from build123d import *

# Parameters (mm, degrees)
F1_DEPTH  = 55
F2_R      = 8
F3_W      = 90
F3_H      = 90
F4_DEPTH  = 15
F5_R      = 8
F6_W      = 15
F6_H      = 10
F7_DEPTH  = 45
F8_R      = 5
F9_W      = 50
F9_H      = 45
F10_DEPTH = 50
F12_DEPTH = 45
F13_W     = 5
F13_H     = 40
F14_DEPTH = 15.001
F16_DEPTH = 5


with BuildPart() as f1:
    # F0 (on Front) → F1 (new body)
    with BuildSketch(Plane.XZ):
        Polygon((0, 18), (0, 0), (70, 0), (70, 45), (50, 45), (50, 20), (30, 20), (30, 45), (10, 45), (2.765372, 18), align=None)
    extrude(amount=-F1_DEPTH)

    # F2
    f2_edges = [f1.edges().sort_by_distance(p)[0] for p in [
        (30, 27.5, 20),
        (50, 27.5, 20),
    ]]
    fillet(f2_edges, radius=F2_R)

    # F3 (on face) → F4 (join)
    with BuildSketch(Plane(origin=(0, 0, 0), x_dir=(1, 0, 0), z_dir=(0, 0, -1))):
        with Locations((35, -25)):
            Rectangle(F3_W, F3_H)
    extrude(amount=F4_DEPTH)

    # F5
    f5_edges = [f1.edges().sort_by_distance(p)[0] for p in [
        (-10, 70, -7.5),
        (80, 70, -7.5),
        (-10, -20, -7.5),
        (80, -20, -7.5),
    ]]
    fillet(f5_edges, radius=F5_R)

    # F6 (on face) → F7 (join, through all)
    with BuildSketch(Plane.XY.offset(45)):
        with Locations((17.5, 60)):
            Rectangle(F6_W, F6_H)
    extrude(amount=-F7_DEPTH)

    # F8
    f8_edges = [f1.edges().sort_by_distance(p)[0] for p in [
        (25, 65, 22.5),
        (10, 65, 22.5),
    ]]
    fillet(f8_edges, radius=F8_R)

    # F9 (on face) → F10 (cut)
    with BuildSketch(Plane.XY.offset(45)):
        with Locations((40, 27.5)):
            Rectangle(F9_W, F9_H)
    extrude(amount=-F10_DEPTH, mode=Mode.SUBTRACT)

    # F11 (on face) → F12 (join)
    with BuildSketch(Plane.XY.offset(-5)):
        with BuildLine():
            Line((30, 50), (15, 50))
            Line((15, 50), (15, 35))
            ThreePointArc((15, 35), (25.606602, 39.393398), (30, 50))
        make_face()
    extrude(amount=F12_DEPTH)

    # F13 (on face) → F14 (cut, through all)
    with BuildSketch(Plane.XY):
        with Locations((-7.5, 35)):
            Rectangle(F13_W, F13_H)
        with Locations((77.5, 15)):
            Rectangle(F13_W, F13_H)
    extrude(amount=-F14_DEPTH, mode=Mode.SUBTRACT)

    # F15 (on face) → F16 (cut)
    with BuildSketch(Plane(origin=(0, 0, -15), x_dir=(1, 0, 0), z_dir=(0, 0, -1))):
        Polygon((0, 5), (60, -65), (60, 5), align=None)
    extrude(amount=-F16_DEPTH, mode=Mode.SUBTRACT)


solid = f1.part
Source: CAD feature listing. Evaluate the final solid. Frame: model axes, mm. A direction names the side the tool comes from. Coordinates: 2 decimals unless noted, no trailing zeros. Loops run counter-clockwise (first coordinate to the right, second up) from the corner with the lowest first, then second, coordinate; pieces in that order, holes last. Notation, with made-up numbers: (2, 57) - (16, 57) arc R18 ccw to (16, 83) - close; hole circle Ø6 at (8.25, 28). An arc over 180 degrees is marked (long way). One line per question, with ' | ' between items.
1) Set-up query: faces 1 (the face through (75, 15, -7)), 2 (the face through (6, 55, 18)), 3 (the face through (50, 52, 37)). Return all of +Z, -Z, +X, -X, +Y, -Y with unobstructed straight access to the full face (end or side cutting, diameter ignored); none if empty.
Report:
face 1: +Z, -Z, +X | face 2: +Z, -X, +Y | face 3: +Z, +Y, -Y
2) First-contact query: P1, Ø4, axis at x = -6.5, z = -9, coming from the -Y side; P2, Ø5, axis at y = 52.5, z = 33, coming from the -X side; P3, Ø4.5, axis at x = 24.5, y = 39, coming from the +Z side. Flat tips, straight axial feed; report the tip coordinate or a pass-through.
Report:
P1: stops at y = -19.6 | P2: stops at x = 6.11 | P3: stops at z = 40
3) Line query: line 1 along Y through (x, z) = (59.5, 18); line 2 along Y through (x, z) = (61, -4.5); line 3 along X through (y, z) = (22, 0.5). Output: solid intervals per line, ascending.
Report:
line 1: y = 0 to 5, 50 to 55 | line 2: y = -20 to 5, 50 to 70 | line 3: x = 0 to 15, 65 to 70
4) Section B-B, the plane x = 67.5. Return loops of the section in (y, z).
Report:
outline: (-20, -15) - (70, -15) - (70, 0) - (55, 0) - (55, 45) - (0, 45) - (0, 0) - (-20, 0) - close
5) Section C-C, the plane z = -1.5. Return loops of the section in (x, y).
Report:
outline: (-10, -12) arc R8 ccw to (-2, -20) - (72, -20) arc R8 ccw to (80, -12) - (80, -5) - (75, -5) - (75, 35) - (80, 35) - (80, 62) arc R8 ccw to (72, 70) - (-2, 70) arc R8 ccw to (-10, 62) - (-10, 55) - (-5, 55) - (-5, 15) - (-10, 15) - close; hole (15, 5) - (65, 5) - (65, 50) - (30, 50) arc R15 cw to (15, 35) - close
6) Pull-direction query (X, two-part tool) for faces 4 (the face through (34, 70, -7)), 5 (the face through (80, -8, -7)), 6 (the face through (51, 50, 15)); classes: released by +X, released by -X, zero draft, split by the parting line, or undercut.
Report:
face 4: zero draft | face 5: released by +X | face 6: undercut
7) Section A-A, the plane z = 12.5. Return loops of the section in (x, y), then the cut area to 3 significant figures.
Report:
outline: (0, 0) - (70, 0) - (70, 55) - (25, 55) - (25, 60) arc R5 ccw to (20, 65) - (15, 65) arc R5 ccw to (10, 60) - (10, 55) - (0, 55) - close; hole (15, 5) - (65, 5) - (65, 50) - (30, 50) arc R15 cw to (15, 35) - close | area: 1,920 mm²
8) Section D-D, the plane y = 25. Return loops of the section in (x, z).
Report:
outline: (-5, -15) - (25.71, -15) - (25.71, -10) - (60, -10) - (60, -15) - (75, -15) - (75, 0) - (70, 0) - (70, 45) - (65, 45) - (65, -5) - (15, -5) - (15, 45) - (10, 45) - (2.77, 18) - (0, 18) - (0, 0) - (-5, 0) - close
